from build123d import *

# Parameters (mm, degrees)
CROQUIS2_R              = 3
SALIENTE_EXTRUIR1_DEPTH = 12.7


with BuildPart() as part:
    # Croquis2 → Saliente-Extruir1 (new body)
    with BuildSketch(Plane.XY):
        with BuildLine():
            Line((3.587738838, 0), (39.406158703, 0))
            ThreePointArc((39.406158703, 0), (39.918259557, 0.141074674), (40.285871489, 0.524494569))
            add(Edge.make_bspline(
                [(40.285871489, 0.524494569), (46.911013433, 12.781393637), (50.153045093, 25.954013269), (50, 40)],
                knots=[0.014077908, 0.014077908, 0.014077908, 0.014077908, 1, 1, 1, 1], degree=3))
            ThreePointArc((50, 40), (45, 45), (40, 40))
            add(Edge.make_bspline(
                [(3.057834867, 1.848057652), (18.658480945, 11.5960321), (31.500499666, 23.937674405), (40, 40)],
                knots=[0.060556777, 0.060556777, 0.060556777, 0.060556777, 1, 1, 1, 1], degree=3))
            ThreePointArc((3.057834867, 1.848057652), (2.626474657, 0.724371311), (3.587738838, 0))
        make_face()
        with Locations((45, 40)):
            Circle(CROQUIS2_R, mode=Mode.SUBTRACT)
        with BuildLine():
            Line((15.790154488, 6.97430828), (28.020474624, 18.185435072))
            ThreePointArc((28.020474624, 18.185435072), (29.74708418, 18.675625391), (31.171552095, 17.583673804))
            Line((31.171552095, 17.583673804), (36.607249933, 6.372547013))
            ThreePointArc((36.607249933, 6.372547013), (36.502480714, 4.438184109), (34.807621719, 3.5))
            Line((34.807621719, 3.5), (17.141603745, 3.5))
            ThreePointArc((17.141603745, 3.5), (15.277654099, 4.774953988), (15.790154488, 6.97430828))
        make_face(mode=Mode.SUBTRACT)
        with BuildLine():
            Line((37.307061828, 12.742351686), (33.200366798, 21.212410186))
            ThreePointArc((33.200366798, 21.212410186), (33.110481788, 22.740502603), (34.127447999, 23.884585413))
            Line((34.127447999, 23.884585413), (42.639921091, 28.011845094))
            ThreePointArc((42.639921091, 28.011845094), (44.843064134, 27.705372666), (45.400338187, 25.551954395))
            Line((45.400338187, 25.551954395), (40.994560126, 12.954636215))
            ThreePointArc((40.994560126, 12.954636215), (39.221637148, 11.61820464), (37.307061828, 12.742351686))
        make_face(mode=Mode.SUBTRACT)
    extrude(amount=SALIENTE_EXTRUIR1_DEPTH)


solid = part.part
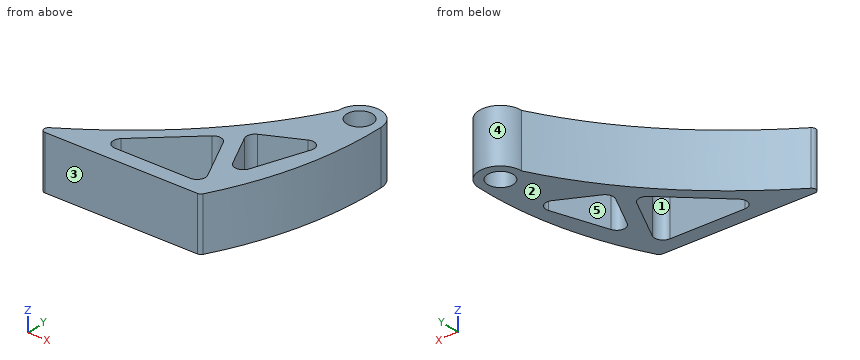
Could you check a few things on this model? Use its own coordinates, in mm. Face numbers are marked on the shaded views. A direction names the side the tool comes from. Give positions to 0.01 mm unless a question says otherwise; leave off trailing zeros. Return JSON: item names as keys, results as strings. Group by question number.
Q1. Please list where these lines run through material, in increasing order: line 1 along Y through (x, z) = (35, 11.75); line 2 along X through (y, z) = (16, 10); line 3 along X through (y, z) = (20, 8.5). Write a range as [from, to].
Q2. Thinking about a two-plate mould opening in Y: for the marked faces 1, 2 and 3, which applies, pulls with the +Y half, pulls with the -Y half, needs draft (parallel to the pull), parting line crosses it, or undercut?
Q3. Will these pins go through, and if not, where does the flat tip stop? pin 1 Ø6 at (y, z) = (11, 10.5) entering from -X; pin 2 Ø1 at (x, z) = (40, 3) entering from -Y.
Q4. Suppose I cut it at A-A, the plane z = 1.5. State how many separate pieces and enclosed holes the cut face has, and give its area (3 significant figures).
Q5. Which directions (+Z, -Z, +X, -X, +Y, -Y) give clear straight access to the entire face, cutting with the end or side of a thin tool? Please do the marked faces 4 and 5.
Resolved:
{
 "1": {"line 1": "y = [0, 3.51], [9.69, 17.5], [24.31, 31.69]", "line 2": "x = [21.58, 25.64], [31.94, 35.73], [42.06, 46.71]", "line 3": "x = [25.59, 33.79], [43.46, 47.78]"},
 "2": {"face 1": "undercut", "face 2": "needs draft", "face 3": "pulls with the -Y half"},
 "3": {"pin 1": "stops at x = 12.05", "pin 2": "stops at y = 0"},
 "4": {"separate pieces": "1", "enclosed holes": "3", "area": "606 mm2"},
 "5": {"face 4": "+Z, -Z, +Y", "face 5": "+Z, -Z"}
}
